Geometry: final body of the model. Coordinates: model frame, mm. A direction names the side the tool comes from. Give positions to 0.01 mm unless a question says otherwise; leave off trailing zeros. Write each loop counter-clockwise with the first axis right and the second up, starting at its lowest first coordinate (ties: lowest second). Pieces come first, ordered by that corner, then holes.
Q1. Section B-B (y = 22.85). Return the cut outline in (x, z).
Q2. Section C-C (z = 1.75). Return the cut outline in (x, y).
Q3. Mould query, pull axis Y, two halves, no side actions, for faces 1 (the flat face through (0, 117, 0)), 2 (the flat face through (-25, 64, 0)), 3 (the flat face through (0, 0, 0)), 4 (the flat face through (0, 140, 0)). Classes: +Y half, -Y half, draft (parallel to the pull), parting line (faces both ways), or undercut.
Q4. Line query: line 1 (Y direction, x = -2, z = 0); line 2 (Y direction, x = 15.5, z = -3); line 3 (Y direction, x = 16.5, z = 4.25). Output: solid intervals per line, ascending.
Q5. Section A-A (x = -4.5). Return the cut outline in (y, z).
Q6. Reachability of faces 5 (the flat face through (0, 102, 0)), 6 (the flat face through (-20, 135, 0)) from +Z, -Z, +X, -X, +Y, -Y: full face, straight path, thin tool, end or side. Return the list, or none.
from build123d import *

# Parameters (mm, degrees)
SKETCH1_W           = 50
SKETCH1_H           = 140
SKETCH1_R           = 2.5
SKETCH1_W_2         = 10
SKETCH1_H_2         = 5
BOSS_EXTRUDE1_DEPTH = 5
CHAMFER1_SIZE       = 10


with BuildPart() as part:
    # Sketch1 → Boss-Extrude1 (new, symmetric)
    with BuildSketch(Plane.XY):
        with Locations((0, 70)):
            Rectangle(SKETCH1_W, SKETCH1_H)
        with Locations((-16, 22.85)):
            Circle(SKETCH1_R, mode=Mode.SUBTRACT)
        with Locations((15.5, 22.85)):
            Circle(SKETCH1_R, mode=Mode.SUBTRACT)
        with Locations((-5, 102.5)):
            Rectangle(SKETCH1_W_2, SKETCH1_H_2, mode=Mode.SUBTRACT)
        with Locations((-5, 117.5)):
            Rectangle(SKETCH1_W_2, SKETCH1_H_2, mode=Mode.SUBTRACT)
    extrude(amount=BOSS_EXTRUDE1_DEPTH, both=True)

    # Chamfer1
    chamfer1_edges = [part.edges().sort_by_distance(p)[0] for p in [
        (25, 140, 0),
        (-25, 140, 0),
    ]]
    chamfer(chamfer1_edges, length=CHAMFER1_SIZE)


solid = part.part
Computed:
1. outline: (-25, -5) - (-18.5, -5) - (-18.5, 5) - (-25, 5) - close; (-13.5, -5) - (13, -5) - (13, 5) - (-13.5, 5) - close; (18, -5) - (25, -5) - (25, 5) - (18, 5) - close
2. outline: (-25, 0) - (25, 0) - (25, 130) - (15, 140) - (-15, 140) - (-25, 130) - close; hole circle Ø5 at (-16, 22.85); hole (-10, 100) - (0, 100) - (0, 105) - (-10, 105) - close; hole (-10, 115) - (0, 115) - (0, 120) - (-10, 120) - close; hole circle Ø5 at (15.5, 22.85)
3. face 1: undercut
3. face 2: draft
3. face 3: -Y half
3. face 4: +Y half
4. line 1: y = 0 to 100, 105 to 115, 120 to 140
4. line 2: y = 0 to 20.35, 25.35 to 139.5
4. line 3: y = 0 to 20.56, 25.14 to 138.5
5. outline: (0, -5) - (100, -5) - (100, 5) - (0, 5) - close; (105, -5) - (115, -5) - (115, 5) - (105, 5) - close; (120, -5) - (140, -5) - (140, 5) - (120, 5) - close
6. face 5: +Z, -Z
6. face 6: +Z, -Z, -X, +Y
